Check sheet for the modelled part. Datum: model origin and axes. Units: mm. A direction names the side the tool comes from. Give positions to 0.01 mm unless a question says otherwise; leave off trailing zeros. Order: outer loops, then holes, each group sorted by start corner. A loop starts at its lowest first (then second) coordinate and runs counter-clockwise, first axis right, second up.
```python
from build123d import *

# Parameters (mm, degrees)
F0_R     = 3.5
F1_DEPTH = 5
F2_R     = 4.5
F3_DEPTH = 1
F4_R     = 2.5
F5_DEPTH = 30
F6_R     = 0.3


with BuildPart() as f1:
    # F0 (on Top) → F1 (new body)
    with BuildSketch(Plane.XY):
        Circle(F0_R)
        Polygon((-2.309401, 0), (-1.154701, 2), (1.154701, 2), (2.309401, 0), (1.154701, -2), (-1.154701, -2), align=None, mode=Mode.SUBTRACT)
    extrude(amount=F1_DEPTH)

    # F2 (on face) → F3 (join)
    with BuildSketch(Plane(origin=(0, 0, 0), x_dir=(1, 0, 0), z_dir=(0, 0, -1))):
        Circle(F2_R)
    extrude(amount=F3_DEPTH)

    # F4 (on face) → F5 (join)
    with BuildSketch(Plane(origin=(0, 0, -1), x_dir=(1, 0, 0), z_dir=(0, 0, -1))):
        Circle(F4_R)
    extrude(amount=F5_DEPTH)

    # F6
    f6_edges = [f1.edges().sort_by_distance(p)[0] for p in [
        (-4.5, 0, 0),
    ]]
    fillet(f6_edges, radius=F6_R)


solid = f1.part
```
(1) Cross-section at A-A on x = 0. Enter the section's corners in (y, z).
Response values:
outline: (-4.5, -1) - (-2.5, -1) - (-2.5, -31) - (2.5, -31) - (2.5, -1) - (4.5, -1) - (4.5, -0.3) arc R0.3 ccw to (4.2, 0) - (3.5, 0) - (3.5, 5) - (2, 5) - (2, 0) - (-2, 0) - (-2, 5) - (-3.5, 5) - (-3.5, 0) - (-4.2, 0) arc R0.3 ccw to (-4.5, -0.3) - close
(2) Gauge pin test, flat ends, axial feed: pin 1 Ø1.5 at (x, z) = (-2, -11) entering from +Y; pin 2 Ø2.5 at (x, z) = (0, 1.5) entering from +Y; pin 3 Ø1.2 at (x, y) = (-0.5, 0.5) entering from +Z. Record the tip position at first contact, or that the pin passes through.
Response values:
pin 1: stops at y = 2.17
pin 2: stops at y = 3.5
pin 3: stops at z = 0
(3) Release check for a two-part mould opening along Y. For faces 4 (the face through (-0.59, -4.46, -0.65)), 5 (the face through (2, -2, 5)), 6 (the face through (1.724, 1.014, 2.465)) record: released by +Y, released by -Y, zero draft, split by the parting line, or undercut.
Response values:
face 4: split by the parting line
face 5: zero draft
face 6: undercut
(4) Material ranges on L1, parallel to Z at x = -2.5, y = -3; L2, parallel to Z at x = 0, y = -3; L3, parallel to Y at x = 0, z = -9.5, recorded low to high.
Response values:
L1: z = -1 to 0
L2: z = -1 to 5
L3: y = -2.5 to 2.5
(5) Cross-section at B-B on z = -17. Enter the section's corners in (x, y).
Response values:
outline: circle Ø5 at (0, 0)
(6) Set-up check for faces 1 (the face through (-0.54, 2.44, -15.79)), 2 (the face through (0, 0, -31)), 3 (the face through (-1.724, -1.014, 2.465)): record each of +Z, -Z, +X, -X, +Y, -Y from which the full face is reachable in a straight line by a thin tool's end or side.
Response values:
face 1: -Z
face 2: -Z, +X, -X, +Y, -Y
face 3: +Z
